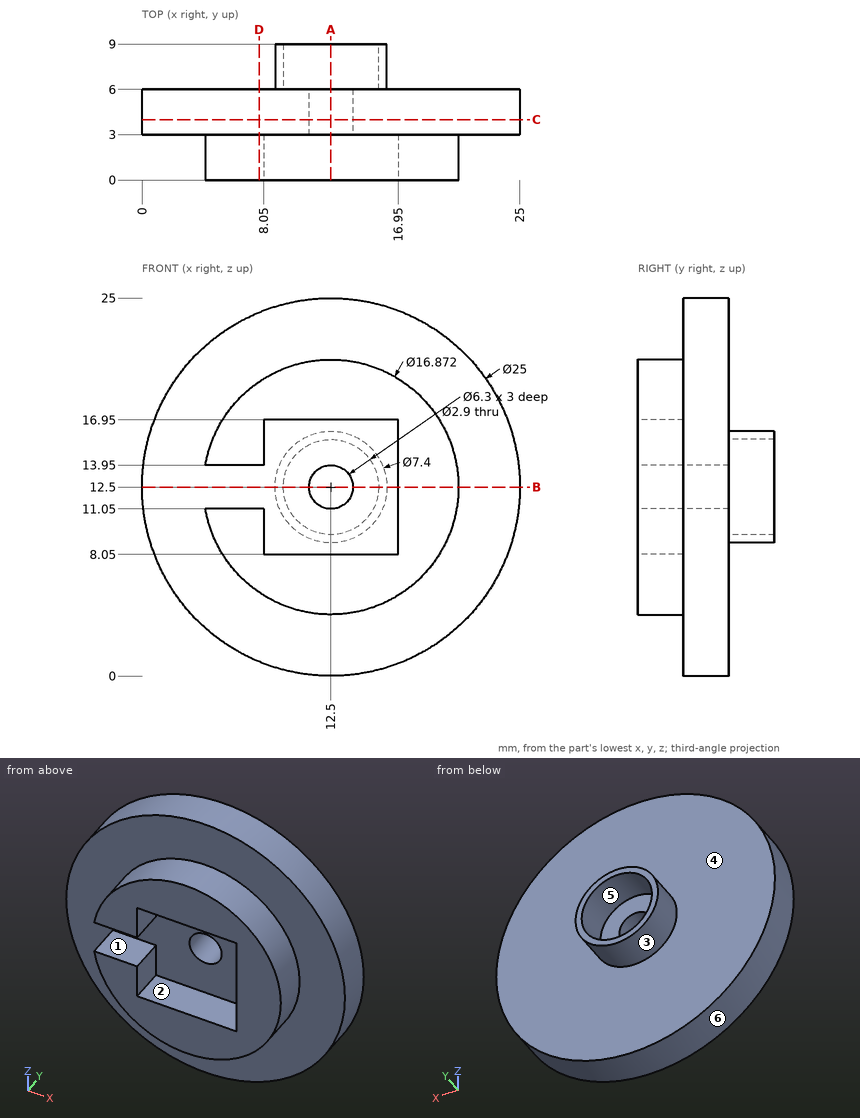
The drawing under review shows one solid part. Ordinate dimensions are in mm from its lowest x, y, z. A direction names the side the tool comes from. Coordinates: 2 decimals unless noted, no trailing zeros. Write each loop counter-clockwise with the first axis right and the second up, starting at its lowest first coordinate (ties: lowest second). Pieces come first, ordered by that corner, then holes. Notation, with made-up numbers: (37.5, -21.5) - (53.5, -21.5) arc R30 cw to (53.5, 0.5) - close; hole circle Ø8 at (79.25, -35.5). An arc over 180 degrees is marked (long way). Put each result on its own line as item: value.
1. Machinability: for the marked faces 1, 2 and 3, which of the approach directions +Z, -Z, +X, -X, +Y, -Y give a long, thin tool a straight path to every point of the face, cutting with its end or side? Answer none if there is none.
Values found:
face 1: -X, -Y
face 2: -Y
face 3: +Y
2. Add section C-C, the plane y = 4. Give the boundary of the cut face in (x, z), then the cut area to 3 significant figures.
Values found:
outline: circle Ø25 at (12.5, 12.5); hole circle Ø2.9 at (12.5, 12.5)
area: 484 mm²
3. Add section B-B, the plane z = 12.5. Give the boundary of the cut face in (x, y).
Values found:
outline: (0, 3) - (11.05, 3) - (11.05, 6) - (9.35, 6) - (9.35, 9) - (8.8, 9) - (8.8, 6) - (0, 6) - close; (13.95, 3) - (16.95, 3) - (16.95, 0) - (20.94, 0) - (20.94, 3) - (25, 3) - (25, 6) - (16.2, 6) - (16.2, 9) - (15.65, 9) - (15.65, 6) - (13.95, 6) - close
4. Mouldability with a two-part tool opening along X and no side actions: class the marked faces 4, 5 and 6 as released by +X, released by -X, zero draft, split by the parting line, or undercut.
Values found:
face 4: zero draft
face 5: undercut
face 6: split by the parting line
5. For pin 1 (5 mm diameter, centred on x = 2.5, y = 7.5, fed in from -Z) (1 decimal); pin 2 (3.5 mm diameter, centred on y = 1, z = 15.5, fed in from +X); pin 3 (3.5 mm diameter, centred on x = 5, y = 1, fed in from +Z); pin 4 (2.5 mm diameter, centred on x = 12.5, z = 12.5, fed in from +Y), all flat-tipped, find the tip position at first contact; note any pin that passes through.
Values found:
pin 1: z = 2.9
pin 2: x = 20.84
pin 3: z = 18.67
pin 4: through
6. Add section D-D, the plane x = 7.75. Give the boundary of the cut face in (y, z).
Values found:
outline: (0, 5.53) - (3, 5.53) - (3, 0.94) - (6, 0.94) - (6, 24.06) - (3, 24.06) - (3, 19.47) - (0, 19.47) - (0, 13.95) - (3, 13.95) - (3, 11.05) - (0, 11.05) - close
7. Add section A-A, the plane x = 12.5. Give the boundary of the cut face in (y, z).
Values found:
outline: (0, 4.06) - (3, 4.06) - (3, 0) - (6, 0) - (6, 8.8) - (9, 8.8) - (9, 9.35) - (6, 9.35) - (6, 11.05) - (3, 11.05) - (3, 8.05) - (0, 8.05) - close; (0, 16.95) - (3, 16.95) - (3, 13.95) - (6, 13.95) - (6, 15.65) - (9, 15.65) - (9, 16.2) - (6, 16.2) - (6, 25) - (3, 25) - (3, 20.94) - (0, 20.94) - close
8. Wall thickness on probe 1 along Z at (x, y) = (12.5, 8.2); probe 2 along Z at (x, y) = (12.5, 4.75): over which ranges is each line inside the solid? List them lowest first.
Values found:
probe 1: 8.8 to 9.35, 15.65 to 16.2
probe 2: 0 to 11.05, 13.95 to 25
